Design review of the part built by this model. Coordinates are the model's own, in mm. Coordinates: 2 decimals unless noted, no trailing zeros. Write each loop counter-clockwise with the first axis right and the second up, starting at its lowest first coordinate (ties: lowest second). Pieces come first, ordered by that corner, then holes.
Q1. Clearance check with flat-ended pins moving along their axes: pin 1 Ø2 at (x, z) = (-47, 3) entering from +Y; pin 2 Ø3 at (x, y) = (15, -11) entering from -Z; pin 3 Ø1.2 at (y, z) = (-11.5, 2.5) entering from -X; pin 4 Ø2 at (x, z) = (42.5, 1.5) entering from +Y. State where each tip first meets the part, or that it passes through.
Q2. Add section B-B, the plane y = 6.5. Give the boundary of the cut face in (x, z).
Q3. Add section C-C, the plane x = 48.5. Give the boundary of the cut face in (y, z), plus the area to 3 significant figures.
Q4. To check wall thickness, follow probe 1 along X at (y, z) = (-12.75, 1.85); probe 2 along X at (y, z) = (1.5, 2.05); probe 3 along Y at (x, z) = (70.5, 1.35). State the ranges of each line that lie inside material, in increasing order.
Q5. Add section A-A, the plane y = -11.5. Give the boundary of the cut face in (x, z), plus the area to 3 significant figures.
Autodesk Inventor part; units mm, degrees
ref_plane "YZ Plane" through (0, 0, 0) normal (1, 0, 0) x (0, 1, 0)
ref_plane "XZ Plane" through (0, 0, 0) normal (0, 1, 0) x (-1, 0, 0)
ref_plane "XY Plane" through (0, 0, 0) normal (0, 0, 1) x (1, 0, 0)
sketch "Sketch1" plane through (0, 0, 0) normal (0, 0, 1) x (1, 0, 0)
  line L0 (-80, 14) -> (80, 14)
  line L1 (80, 14) -> (80, -14)
  line L2 (80, -14) -> (-80, -14)
  line L3 (-80, -14) -> (-80, 14)
  point P0 (0, 0)
  dimension "d0" = 160
  dimension "d1" = 28
  dimension "d2" = 14
  dimension "d3" = 80
extrude "Base" add sketch "Sketch1" along normal blind 4
sketch "Sketch2" plane through (0, 0, 4) normal (0, 0, 1) x (1, 0, 0)
  line L0 (-80, 14) -> (80, 14)
  line L1 (80, -14) -> (-80, -14)
  line L2 (-50, 14) -> (-30, 14)
  line L3 (-30, 14) -> (-30, 10)
  line L4 (-30, 10) -> (-50, 10)
  line L5 (-50, 10) -> (-50, 14)
  line L6 (-10, 14) -> (10, 14)
  line L7 (10, 14) -> (10, 10)
  line L8 (10, 10) -> (-10, 10)
  line L9 (-10, 10) -> (-10, 14)
  line L10 (30, 14) -> (50, 14)
  line L11 (50, 14) -> (50, 10)
  line L12 (50, 10) -> (30, 10)
  line L13 (30, 10) -> (30, 14)
  line L14 (-50, -10) -> (-30, -10)
  line L15 (-30, -10) -> (-30, -14)
  line L16 (-30, -14) -> (-50, -14)
  line L17 (-50, -14) -> (-50, -10)
  line L18 (-10, -10) -> (10, -10)
  line L19 (10, -10) -> (10, -14)
  line L20 (10, -14) -> (-10, -14)
  line L21 (-10, -14) -> (-10, -10)
  line L22 (30, -10) -> (50, -10)
  line L23 (50, -10) -> (50, -14)
  line L24 (50, -14) -> (30, -14)
  line L25 (30, -14) -> (30, -10)
  line L26 (80, 14) -> (80, -14)
  line L27 (-80, -14) -> (-80, 14)
  line L28 (-80, -10) -> (-70, -10)
  line L29 (-70, -10) -> (-70, -14)
  line L30 (-70, -14) -> (-80, -14)
  line L31 (-80, -14) -> (-80, -10)
  line L32 (-80, 14) -> (-70, 14)
  line L33 (-70, 14) -> (-70, 10)
  line L34 (-70, 10) -> (-80, 10)
  line L35 (-80, 10) -> (-80, 14)
  line L36 (70, 14) -> (80, 14)
  line L37 (80, 14) -> (80, 10)
  line L38 (80, 10) -> (70, 10)
  line L39 (70, 10) -> (70, 14)
  line L40 (70, -10) -> (80, -10)
  line L41 (80, -10) -> (80, -14)
  line L42 (80, -14) -> (70, -14)
  line L43 (70, -14) -> (70, -10)
  point P0 (0, 0)
  dimension "d6" = 20
  dimension "d7" = 4
  dimension "d10" = 40
  dimension "d19" = 20
  dimension "d20" = 4
  dimension "d21" = 40
  dimension "d25" = 0
  dimension "d40" = 4
  dimension "d42" = 10
  dimension "d43" = 10
  dimension "d44" = 10
  dimension "d45" = 4
  dimension "d54" = 10
  dimension "d55" = 4
  dimension "d64" = 10
  dimension "d65" = 4
  dimension "d74" = 10
  dimension "d75" = 4
  dimension "d76" = 0
  dimension "d77" = 0
  dimension "d78" = 0
  dimension "d79" = 0
  dimension "d80" = 0
  dimension "d81" = 0
  dimension "d82" = 0
  dimension "d83" = 0
extrude "Platformsleeves" cut sketch "Sketch2" against normal blind 4 contours L0 L33 L34 L27 | L0 L3 L4 L5 | L28 L29 L1 L27 | L0 L7 L8 L9 | L17 L14 L15 L1 | L0 L11 L12 L13 | L21 L18 L19 L1 | L0 L26 L38 L39 | L25 L22 L23 L1 | L26 L1 L43 L40
sketch "Sketch4" plane through (0, 0, 4) normal (0, 0, 1) x (1, 0, 0)
  line L0 (30, 10) -> (30, 14)
  line L1 (-30, 14) -> (-30, 10)
  line L2 (-30, 10) -> (-50, 10)
  line L3 (50, 10) -> (30, 10)
  line L4 (-44, 10) -> (-40, 10)
  line L5 (-40, 10) -> (-40, 0)
  line L6 (-40, 0) -> (-44, 0)
  line L7 (-44, 0) -> (-44, 10)
  line L8 (40, 10) -> (44, 10)
  line L9 (44, 10) -> (44, 0)
  line L10 (44, 0) -> (40, 0)
  line L11 (40, 0) -> (40, 10)
  point P0 (0, 0)
  dimension "d86" = 4
  dimension "d87" = 10
  dimension "d88" = 10
  dimension "d89" = 0
  dimension "d90" = 4
  dimension "d91" = 10
  dimension "d92" = 10
  dimension "d93" = 0
extrude "Sleeves" cut sketch "Sketch4" against normal blind 4
properties part number "LongMiddleStructure"
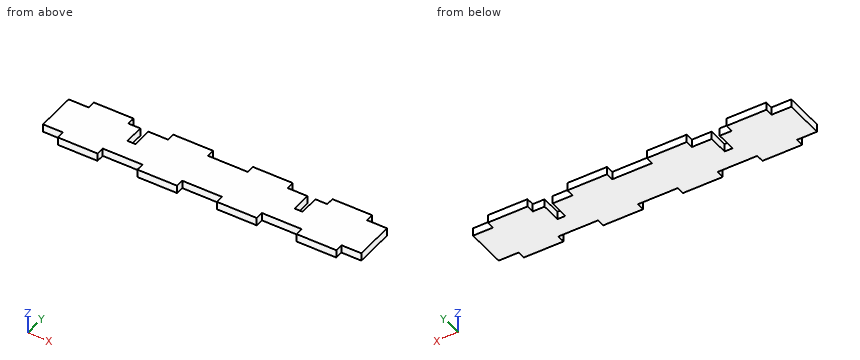
Here are the results:
1. pin 1: stops at y = 10
1. pin 2: stops at z = 0
1. pin 3: stops at x = -70
1. pin 4: stops at y = 0
2. outline: (-80, 0) - (-44, 0) - (-44, 4) - (-80, 4) - close; (-40, 0) - (40, 0) - (40, 4) - (-40, 4) - close; (44, 0) - (80, 0) - (80, 4) - (44, 4) - close
3. outline: (-10, 0) - (10, 0) - (10, 4) - (-10, 4) - close
3. area: 80.0 mm2
4. probe 1: x = -70 to -50, -30 to -10, 10 to 30, 50 to 70
4. probe 2: x = -80 to -44, -40 to 40, 44 to 80
4. probe 3: y = -10 to 10
5. outline: (-70, 0) - (-50, 0) - (-50, 4) - (-70, 4) - close; (-30, 0) - (-10, 0) - (-10, 4) - (-30, 4) - close; (10, 0) - (30, 0) - (30, 4) - (10, 4) - close; (50, 0) - (70, 0) - (70, 4) - (50, 4) - close
5. area: 320 mm2
